Autodesk Inventor part; units mm, degrees
ref_plane "YZ Plane" through (0, 0, 0) normal (1, 0, 0) x (0, 1, 0)
ref_plane "XZ Plane" through (0, 0, 0) normal (0, 1, 0) x (-1, 0, 0)
ref_plane "XY Plane" through (0, 0, 0) normal (0, 0, 1) x (1, 0, 0)
sketch "Sketch1" plane through (0, 0, 0) normal (0, 0, 1) x (1, 0, 0)
  line L0 (0, -30) -> (0, 0)
  line L1 (0, 0) -> (-170, 0)
  line L2 (-170, 0) -> (-170, -15)
  line L3 (-155, -30) -> (-105, -30)
  line L4 (-105, -30) -> (-105, -40)
  arc A0 (-105, -40) -> (0, -30) centre (-80.4998, 258.9979) ccw
  arc A1 (-170, -15) -> (-155, -30) centre (-155, -15) ccw
  circle A2 centre (-155, -15) radius 5
  circle A3 centre (-125, -15) radius 5
  circle A4 centre (-15, -15) radius 5
  point P0 (-170, -30)
  dimension "d0" = 170
  dimension "d1" = 30
  dimension "d2" = 30
  dimension "d3" = 65
  dimension "d4" = 10
  dimension "d6" = 300
  dimension "d7" = 15
  dimension "d8" = 10
  dimension "d9" = 10
  dimension "d10" = 10
  dimension "d11" = 15
  dimension "d12" = 30
  dimension "d13" = 15
  dimension "d14" = 15
extrude "Extrusion1" add sketch "Sketch1" along normal blind 7.9375
chamfer "Chamfer1" distance 7.9375 angle 5 1 edges at (-52.0571, -39.6507, 0) measured on face at (-48.5408, -39.295, 5.2917)
properties part number "Upper blade"
Part model, mm, in its own coordinate system. A direction names the side the tool comes from. Give positions to 0.01 mm unless a question says otherwise; leave off trailing zeros. Order: outer loops, then holes, each group sorted by start corner. A loop starts at its lowest first (then second) coordinate and runs counter-clockwise, first axis right, second up. Notation, with made-up numbers: M 52,14 L 64,14 A26 ccw 64,29 Z; hole C 43,53 d2. An arc over 180 degrees is marked long. Use a Markdown table: item, result. Add a question column.
(1) Mould opens along Y. For faces 3 (the face through (-159, -12, 4)), 4 (the face through (-86, -15, 0)), 5 (the face through (-165.49, -25.72, 3.91)) say: +Y half, -Y half, draft (parallel to the pull), parting line (faces both ways), or undercut.
(2) Saw through at B-B, the plane z = 2.75. Give the cut face in (x, y), and give its area (3 significant figures).
(3) Probe line 1 along X through (y, z) = (-13.5, 3.5); line 2 along Y through (x, z) = (-125, 6.75); line 3 along X through (y, z) = (-11, 7). List the from-to ranges inside material, lowest first. Write a range as [from, to].
(4) Drop a flat-ended pin along its axis: P1, Ø2, axis at y = -22, z = 3, coming from the -X side. Give the stop position or say it passes through.
(5) Saw through at A-A, the plane x = -125. Give the cut face in (y, z).
(6) 3-axis set-ups, long thin cutter, end or side, ignore diameter. For faces 1 (the face through (0, -15, 4)), 2 (the face through (-130, -30, 4)): which of +Z, -Z, +X, -X, +Y, -Y reach the whole face in a straight line?
Answer key:
| question | item | result |
|---|---|---|
| 1 | face 3 | undercut |
| 1 | face 4 | draft |
| 1 | face 5 | -Y half |
| 2 | outline | M -170,-15 A15 ccw -155,-30 L -105,-30 L -105,-39.54 A299.55 ccw 0,-29.53 L 0,0 L -170,0 Z; hole C -155,-15 d10; hole C -125,-15 d10; hole C -15,-15 d10 |
| 2 | area | 5,620 mm^2 |
| 3 | line 1 | [-170, -159.77], [-150.23, -129.77], [-120.23, -19.77], [-10.23, 0] |
| 3 | line 2 | [-30, -20], [-10, 0] |
| 3 | line 3 | [-170, -158], [-152, -128], [-122, -18], [-12, 0] |
| 4 | P1 | x = -168.75 |
| 5 | outline | M -30,0 L -20,0 L -20,7.94 L -30,7.94 Z; M -10,0 L 0,0 L 0,7.94 L -10,7.94 Z |
| 6 | face 1 | +Z, -Z, +X, +Y, -Y |
| 6 | face 2 | +Z, -Z, -X, -Y |
